The figure shows three views and two pictorial views of one solid part (mm, origin at its lowest corner). Answer the questions. A direction names the side the tool comes from. Round coordinates to 2 decimals unless told otherwise and drop trailing zeros. Write each loop counter-clockwise with the first axis right and the second up, starting at its lowest first coordinate (ties: lowest second). Pieces come first, ordered by that corner, then holes.
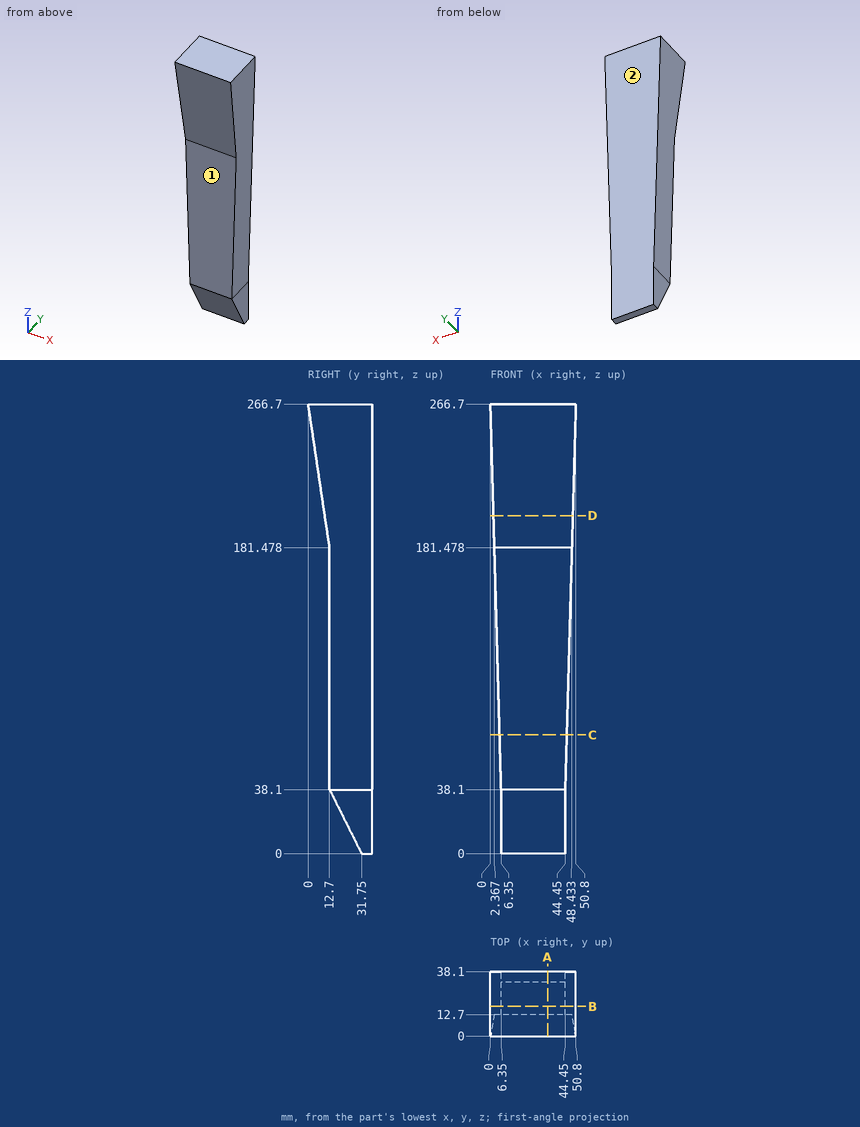
Q1. Straight lines are drawn through the part: probe 1 along Y at (x, z) = (23, 159); probe 2 along X at (y, z) = (24.5, 23); probe 3 along X at (y, z) = (22, 183) (1 decimal). For each, find the intervals that lie inside material, in ascending order.
Verdict:
probe 1: y = 12.7 to 38.1
probe 2: x = 6.35 to 44.45
probe 3: x = 2.3 to 48.5
Q2. Which of the six approach directions +Z, -Z, +X, -X, +Y, -Y give full straight-line access (tool end or side, diameter ignored) to the marked faces 1 and 2?
Verdict:
face 1: -Z, +X, -X, -Y
face 2: +Z, -Z, +X, -X, +Y
Q3. Section D-D (z = 200.5) is taken. Determine the outline of the cut face in (x, y) (1 decimal), then the cut area to 3 significant figures.
Verdict:
outline: (1.8, 9.9) - (49, 9.9) - (49, 38.1) - (1.8, 38.1) - close
area: 1,330 mm2
Q4. Section C-C (z = 70.5) is taken. Determine the outline of the cut face in (x, y).
Verdict:
outline: (5.45, 12.7) - (45.35, 12.7) - (45.35, 38.1) - (5.45, 38.1) - close
Q5. Flat-ended cylindrical pins translate along their axes: pin 1 Ø4 at (y, z) = (10.5, 184.5) entering from +X; pin 2 Ø8 at (y, z) = (11.5, 224) entering from -X (3 decimals); pin 3 Ø1 at (x, y) = (17, 21) entering from -Z; pin 4 Ø6 at (x, y) = (16, 33.5) entering from -Z. Find the tip coordinate at first contact, or state that the pin passes through.
Verdict:
pin 1: stops at x = 48.55
pin 2: stops at x = 1.075
pin 3: stops at z = 20.5
pin 4: stops at z = 0
Q6. Section A-A (x = 34) is taken. Determine the outline of the cut face in (y, z), then the cut area to 3 significant figures.
Verdict:
outline: (0, 266.7) - (12.7, 181.48) - (12.7, 38.1) - (31.75, 0) - (38.1, 0) - (38.1, 266.7) - close
area: 6,950 mm2
Q7. Section B-B (y = 17.5) is taken. Determine the outline of the cut face in (x, z), then the cut area to 3 significant figures.
Verdict:
outline: (0, 266.7) - (6.35, 38.1) - (6.35, 28.5) - (44.45, 28.5) - (44.45, 38.1) - (50.8, 266.7) - close
area: 10,500 mm2
